```python
from build123d import *

# Parameters (mm, degrees)
SKETCH1_W               = 323
SKETCH1_H               = 45.34
BOSS_EXTRUDE1_DEPTH     = 3
SKETCH2_W               = 71
SKETCH2_H               = 24.5
SKETCH2_R               = 13.5
SKETCH2_W_2             = 28
SKETCH2_H_2             = 31
SKETCH2_R_2             = 5.8
SKETCH2_R_3             = 1.75
CUT_EXTRUDE1_DEPTH      = 1
CUT_EXTRUDE1_DEPTH_BACK = 4
SKETCH3_R               = 1.5
SKETCH3_W               = 43
SKETCH3_H               = 7
CUT_EXTRUDE2_DEPTH      = 10
CUT_EXTRUDE4_DEPTH      = 10
SKETCH6_W               = 3
SKETCH6_H               = 45.34
CUT_EXTRUDE5_DEPTH      = 10
SKETCH7_R               = 1.5
CUT_EXTRUDE6_DEPTH      = 4


with BuildPart() as part:
    # Sketch1 → Boss-Extrude1 (new body)
    with BuildSketch(Plane.XY):
        Rectangle(SKETCH1_W, SKETCH1_H)
    extrude(amount=BOSS_EXTRUDE1_DEPTH)

    # Sketch2 → Cut-Extrude1 (cut, two sides)
    with BuildSketch(Plane.XY.offset(3)) as cut_extrude1_sk:
        with Locations((-101, 0)):
            Rectangle(SKETCH2_W, SKETCH2_H)
        Polygon((-61, 2.2), (-65.5, 6.6), (-65.5, -6.6), (-61, -2.2), align=None)
        with Locations((-39.75, 0)):
            Circle(SKETCH2_R)
        Rectangle(SKETCH2_W_2, SKETCH2_H_2)
        with Locations((44, 0)):
            Circle(SKETCH2_R_2)
        with Locations((44, 15.67)):
            Circle(SKETCH2_R_3)
        with Locations((74, 0)):
            Circle(SKETCH2_R_3)
        with Locations((104, 0)):
            Circle(SKETCH2_R_3)
        with Locations((119, 0)):
            Circle(SKETCH2_R_3)
        with Locations((134, 0)):
            Circle(SKETCH2_R_3)
    extrude(amount=CUT_EXTRUDE1_DEPTH, mode=Mode.SUBTRACT)
    extrude(cut_extrude1_sk.sketch, amount=-CUT_EXTRUDE1_DEPTH_BACK, mode=Mode.SUBTRACT)

    # Sketch3 → Cut-Extrude2 (cut)
    with BuildSketch(Plane(origin=(0, 0, 0), x_dir=(-1, 0, 0), z_dir=(0, 0, -1))):
        with Locations((63.2, 16.55)):
            Circle(SKETCH3_R)
        with Locations((63.2, -15.05)):
            Circle(SKETCH3_R)
        with Locations((138.8, -15.05)):
            Circle(SKETCH3_R)
        with Locations((138.8, 16.55)):
            Circle(SKETCH3_R)
        with Locations((155.5, 16.55)):
            Circle(SKETCH3_R)
        with Locations((155.5, -15.05)):
            Circle(SKETCH3_R)
        with Locations(Location((-155.5, -15.05, 0), (0, 0, 180))):  # turned: the seam where the file's is
            Circle(SKETCH3_R)
        with Locations(Location((-155.5, 16.55, 0), (0, 0, 180))):  # turned: the seam where the file's is
            Circle(SKETCH3_R)
        with Locations((114.3, 15.25)):
            Rectangle(SKETCH3_W, SKETCH3_H)
    extrude(amount=-CUT_EXTRUDE2_DEPTH, mode=Mode.SUBTRACT)

    # Sketch5 → Cut-Extrude4 (cut)
    with BuildSketch(Plane.XY.offset(3)):
        with BuildLine():
            ThreePointArc((18.6, -1.25), (19.85, 0), (18.6, 1.25))
            ThreePointArc((18.6, 1.25), (17.35, 0), (18.6, -1.25))
        make_face()
        with BuildLine():
            ThreePointArc((-18.6, -1.25), (-17.35, 0), (-18.6, 1.25))
            ThreePointArc((-18.6, 1.25), (-19.85, 0), (-18.6, -1.25))
        make_face()
    extrude(amount=-CUT_EXTRUDE4_DEPTH, mode=Mode.SUBTRACT)

    # Sketch6 → Cut-Extrude5 (cut)
    with BuildSketch(Plane.XY.offset(3)):
        with Locations((-160, 0)):
            Rectangle(SKETCH6_W, SKETCH6_H)
        with Locations((160, 0)):
            Rectangle(SKETCH6_W, SKETCH6_H)
    extrude(amount=-CUT_EXTRUDE5_DEPTH, mode=Mode.SUBTRACT)

    # Sketch7 → Cut-Extrude6 (cut, through all)
    with BuildSketch(Plane(origin=(0, 0, 0), x_dir=(-1, 0, 0), z_dir=(0, 0, -1))):
        with Locations((28.15, -12)):
            Circle(SKETCH7_R)
        with Locations((47.65, -12)):
            Circle(SKETCH7_R)
        with Locations((47.65, 14)):
            Circle(SKETCH7_R)
        with Locations((28.15, 14)):
            Circle(SKETCH7_R)
    extrude(amount=-CUT_EXTRUDE6_DEPTH, mode=Mode.SUBTRACT)


solid = part.part
```
Geometry: final body of the model. Coordinates: model frame, mm. Round coordinates to 2 decimals unless told otherwise and drop trailing zeros. Write each loop counter-clockwise with the first axis right and the second up, starting at its lowest first coordinate (ties: lowest second). Pieces come first, ordered by that corner, then holes. Notation, with made-up numbers: (74.25, 55.25) -> (131.25, 55.25) arc R14 ccw to (131.25, 67.25) -> close; hole circle Ø4 at (8, -15.75). An arc over 180 degrees is marked (long way). Use CSV: the item, a comma, the result in double quotes. Start each with the question number.
Q1. First-contact query: pin 1 Ø2 at (x, y) = (-18.6, 0) entering from -Z. Flat tip, straight axial feed; report the tip coordinate or a pass-through.
Q2. Pull-direction query (Z, two-part tool) for faces 1 (the face through (33, 0, 0)), 2 (the face through (38.206, 0.255, 1.521)), 3 (the face through (33, 0, 3)); classes: pulls with the +Z half, pulls with the -Z half, needs draft (parallel to the pull), parting line crosses it, or undercut.
Q3. Line query: L1, parallel to X at y = -14.5, z = 1.05; L2, parallel to Y at x = -41, z = 0.4; L3, parallel to Y at x = -107, z = 2.4. Output: solid intervals per line, ascending.
Q4. Section B-B (z = 0.75). Give the number of separate pieces and of enclosed holes in the cut face, plus the area to 3 significant figures.
Q5. Section A-A (x = -73.5). Return loops of the section in (y, z), plus the area to 3 significant figures.
Result sheet:
1,pin 1,"through"
2,face 1,"pulls with the -Z half"
2,face 2,"needs draft"
2,face 3,"pulls with the +Z half"
3,L1,"-158.5 to -156.9, -154.1 to -140.2, -137.4 to -64.6, -61.8 to -14, 14 to 154.1, 156.9 to 158.5"
3,L2,"-22.67 to -13.44, 13.44 to 22.67"
3,L3,"-22.67 to -12.25, 18.75 to 22.67"
4,separate pieces,"1"
4,enclosed holes,"22"
4,area,"10,600 mm²"
5,outline,"(-22.67, 0) -> (-12.25, 0) -> (-12.25, 3) -> (-22.67, 3) -> close; (12.25, 0) -> (22.67, 0) -> (22.67, 3) -> (12.25, 3) -> close"
5,area,"62.5 mm²"
